Input: part model. Units: mm. Frame: model coordinates. Coordinates: 2 decimals unless noted, no trailing zeros. Write each loop counter-clockwise with the first axis right and the second up, starting at its lowest first coordinate (ties: lowest second). Pieces come first, ordered by that corner, then holes. Notation, with made-up numbers: (-9, -17.75) -> (28, -17.75) arc R23 cw to (28, -5.75) -> close; hole circle Ø9 at (-7.75, -20.5). An arc over 180 degrees is marked (long way). Use one line per item in the form item = value. Start each with the question number.
(1) Cut plane B-B on y = -1.5. Return the cut outline in (x, z), plus the area to 3 significant figures.
(2) First-contact query: pin 1 (1.8 mm diameter, centred on x = 1.5, y = 1, fed in from +Z); pin 2 (5 mm diameter, centred on x = -3, z = -53.5, fed in from +Y); pin 3 (5 mm diameter, centred on y = -1.5, z = -48.5, fed in from +X). Flat tips, straight axial feed; report the tip coordinate or a pass-through.
(3) Ray query, line 1 along Y through (x, z) = (0, -0.3); line 2 along Z through (x, y) = (-1, -3.25); line 3 along Z through (x, y) = (2, 0). Return the intervals inside material, ascending.
(4) Cut plane A-A on z = -31. Return the cut outline in (x, y), plus the area to 3 significant figures.
```python
from build123d import *

# Parameters (mm, degrees)
SKETCH2_R           = 0.5
BOSS_EXTRUDE1_DEPTH = 100


with BuildPart() as part:
    # Sketch1 → Revolve1 (revolve)
    with BuildSketch(Plane(origin=(0, 0, 0), x_dir=(0, 0, -1), z_dir=(1, 0, 0)), mode=Mode.PRIVATE) as revolve1_sk:
        Polygon((0, 4.5), (0, 3), (0.55, 3), (0.55, 0), (23.25, 0), (23.25, 4.4), (5, 4.4), (5, 4.5), align=None)
    revolve(revolve1_sk.sketch.rotate(Axis((0, 0, 0), (0, 0, 1)), 90), axis=Axis((0, 0, 0), (0, 0, 1)))  # turned: the seam where the file's is

    # Sketch2 → Boss-Extrude1 (add)
    with BuildSketch(Plane(origin=(0, 0, -23.25), x_dir=(-1, 0, 0), z_dir=(0, 0, -1))):
        with Locations((-0.6, 0)):
            Circle(SKETCH2_R)
    boss_extrude1 = extrude(amount=BOSS_EXTRUDE1_DEPTH)

    # Mirror1: Boss-Extrude1 across plane
    add(boss_extrude1.mirror(Plane(origin=(0, 0, 0), x_dir=(0, 0, 1), z_dir=(1, 0, 0))))


solid = part.part
```
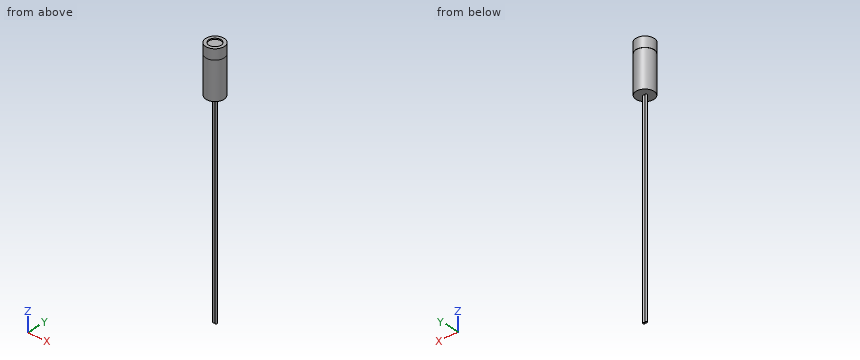
Values:
q1.outline = (-4.24, -5) -> (-4.14, -5) -> (-4.14, -23.25) -> (4.14, -23.25) -> (4.14, -5) -> (4.24, -5) -> (4.24, 0) -> (2.6, 0) -> (2.6, -0.55) -> (-2.6, -0.55) -> (-2.6, 0) -> (-4.24, 0) -> close
q1.area = 191 mm2
q2.pin_1 = -0.55
q2.pin_2 = 0.5
q2.pin_3 = 1.1
q3.line_1 = -4.5 to -3, 3 to 4.5
q3.line_2 = -23.25 to 0
q3.line_3 = -23.25 to -0.55
q4.outline = circle Ø1 at (-0.6, 0); circle Ø1 at (0.6, 0)
q4.area = 1.57 mm2
